The model under review builds one solid part; all positions refer to its coordinate system, in mm. A direction names the side the tool comes from. Give positions to 0.01 mm unless a question says otherwise; leave off trailing zeros. Order: outer loops, then holes, each group sorted by start corner. A loop starts at its lowest first (then second) coordinate and runs counter-clockwise, first axis right, second up. Notation, with made-up numbers: (58.5, 8) - (66.5, 8) arc R20 ccw to (66.5, 25) - close; hole circle Ø5 at (-19.5, -37). An arc over 180 degrees is marked (long way). Answer as CSV lines item,"result". Start each with the question number.
from build123d import *

# Parameters (mm, degrees)
SKIZZE1_W                       = 89
SKIZZE1_H                       = 71.5
LINEAR_AUSTRAGEN1_DEPTH         = 46
SKIZZE12_W                      = 89
SKIZZE12_H                      = 40.19389994
LINEAR_AUSTRAGEN2_DEPTH         = 45
LINEAR_AUSTRAGEN3_DEPTH         = 25
LINEAR_AUSTRAGEN9_DEPTH         = 1.5
SCHNITT_LINEAR_AUSTRAGEN1_DEPTH = 0.5
SKIZZE3_R                       = 1.5
SKIZZE3_R_2                     = 2.15
SKIZZE3_R_3                     = 3.2
LINEAR_AUSTRAGEN4_DEPTH         = 47
SKIZZE4_R                       = 4
SKIZZE4_R_2                     = 5.5
LINEAR_AUSTRAGEN5_DEPTH         = 6.5
SKIZZE13_R                      = 2.5
LINEAR_AUSTRAGEN8_DEPTH         = 8
SKIZZE10_R                      = 3.15
LINEAR_AUSTRAGEN6_DEPTH         = 28.3
SKIZZE11_R                      = 5.5
LINEAR_AUSTRAGEN7_DEPTH         = 23.3
LINEAR_AUSTRAGEN10_DEPTH        = 71.5


with BuildPart() as part:
    # Skizze1 → Linear austragen1 (new body)
    with BuildSketch(Plane.XY):
        with Locations((-3, 35.75)):
            Rectangle(SKIZZE1_W, SKIZZE1_H)
    extrude(amount=LINEAR_AUSTRAGEN1_DEPTH)

    # Skizze12 → Linear austragen2 (cut)
    with BuildSketch(Plane(origin=(0, 71.5, 0), x_dir=(1, 0, 0), z_dir=(0, 1, 0))):
        with Locations((-3, -32.09694997)):
            Rectangle(SKIZZE12_W, SKIZZE12_H)
    extrude(amount=-LINEAR_AUSTRAGEN2_DEPTH, mode=Mode.SUBTRACT)

    # Skizze2 → Linear austragen3 (cut)
    with BuildSketch(Plane.XZ.offset(-26.5)):
        with BuildLine():
            Line((-43.15, 46), (37.15, 46))
            Line((37.15, 46), (37.15, 44.3))
            ThreePointArc((37.15, 44.3), (36.388795325, 40.473165676), (34.221067812, 37.228932188))
            Line((34.221067812, 37.228932188), (28.221067812, 31.228932188))
            ThreePointArc((28.221067812, 31.228932188), (24.976834324, 29.061204675), (21.15, 28.3))
            Line((21.15, 28.3), (-27.15, 28.3))
            ThreePointArc((-27.15, 28.3), (-30.976834324, 29.061204675), (-34.221067812, 31.228932188))
            Line((-34.221067812, 31.228932188), (-40.221067812, 37.228932188))
            ThreePointArc((-40.221067812, 37.228932188), (-42.388795325, 40.473165676), (-43.15, 44.3))
            Line((-43.15, 44.3), (-43.15, 46))
        make_face()
    extrude(amount=LINEAR_AUSTRAGEN3_DEPTH, mode=Mode.SUBTRACT)

    # Skizze14 → Linear austragen9 (cut)
    with BuildSketch(Plane(origin=(0, 1.5, 0), x_dir=(-1, 0, 0), z_dir=(0, 1, 0))):
        with BuildLine():
            Line((13.462912018, 36.3), (33.15, 36.3))
            ThreePointArc((33.15, 36.3), (38.806854249, 38.643145751), (41.15, 44.3))
            Line((41.15, 44.3), (41.15, 46))
            Line((41.15, 46), (-35.15, 46))
            Line((-35.15, 46), (-35.15, 44.3))
            ThreePointArc((-35.15, 44.3), (-32.806854249, 38.643145751), (-27.15, 36.3))
            Line((-27.15, 36.3), (-13.462912018, 36.3))
            ThreePointArc((-13.462912018, 36.3), (0, 33.8), (13.462912018, 36.3))
        make_face()
    extrude(amount=-LINEAR_AUSTRAGEN9_DEPTH, mode=Mode.SUBTRACT)

    # Skizze16 → Schnitt-Linear austragen1 (cut)
    with BuildSketch(Plane(origin=(0, 1.5, 0), x_dir=(1, 0, 0), z_dir=(0, 1, 0))):
        with BuildLine():
            Line((21.15, -28.3), (-27.15, -28.3))
            ThreePointArc((-27.15, -28.3), (-30.976834324, -29.061204675), (-34.221067812, -31.228932188))
            Line((-34.221067812, -31.228932188), (-40.221067812, -37.228932188))
            ThreePointArc((-40.221067812, -37.228932188), (-41.635281374, -40.057359313), (-41.069595949, -43.16862915))
            ThreePointArc((-41.069595949, -43.16862915), (-38.391613931, -38.25636836), (-33.15, -36.3))
            Line((-33.15, -36.3), (-13.462912018, -36.3))
            ThreePointArc((-13.462912018, -36.3), (0, -33.8), (13.462912018, -36.3))
            Line((13.462912018, -36.3), (27.15, -36.3))
            ThreePointArc((27.15, -36.3), (32.391613931, -38.25636836), (35.069595949, -43.16862915))
            ThreePointArc((35.069595949, -43.16862915), (35.635281374, -40.057359313), (34.221067812, -37.228932188))
            Line((34.221067812, -37.228932188), (28.221067812, -31.228932188))
            ThreePointArc((28.221067812, -31.228932188), (24.976834324, -29.061204675), (21.15, -28.3))
        make_face()
    extrude(amount=-SCHNITT_LINEAR_AUSTRAGEN1_DEPTH, mode=Mode.SUBTRACT)

    # Skizze3 → Linear austragen4 (cut, through all)
    with BuildSketch(Plane(origin=(0, 0, 0), x_dir=(-1, 0, 0), z_dir=(0, 0, -1))):
        with Locations((15, 39)):
            Circle(SKIZZE3_R)
        with Locations((-15, 39)):
            Circle(SKIZZE3_R)
        with Locations((25, 64)):
            Circle(SKIZZE3_R_2)
        with Locations((-25, 64)):
            Circle(SKIZZE3_R_3)
    extrude(amount=-LINEAR_AUSTRAGEN4_DEPTH, mode=Mode.SUBTRACT)

    # Skizze4 → Linear austragen5 (cut)
    with BuildSketch(Plane(origin=(0, 0, 12), x_dir=(-1, 0, 0), z_dir=(0, 0, -1))):
        with Locations((25, 64)):
            Circle(SKIZZE4_R)
        with Locations((-25, 64)):
            Circle(SKIZZE4_R_2)
    extrude(amount=LINEAR_AUSTRAGEN5_DEPTH, mode=Mode.SUBTRACT)

    # Skizze13 → Linear austragen8 (cut)
    with BuildSketch(Plane.XY.offset(12)):
        with Locations((15, 39)):
            Circle(SKIZZE13_R)
        with Locations((-15, 39)):
            Circle(SKIZZE13_R)
    extrude(amount=-LINEAR_AUSTRAGEN8_DEPTH, mode=Mode.SUBTRACT)

    # Skizze10 → Linear austragen6 (cut)
    with BuildSketch(Plane(origin=(0, 0, 0), x_dir=(-1, 0, 0), z_dir=(0, 0, -1))):
        with Locations((0, 9.5)):
            Circle(SKIZZE10_R)
    extrude(amount=-LINEAR_AUSTRAGEN6_DEPTH, mode=Mode.SUBTRACT)

    # Skizze11 → Linear austragen7 (cut)
    with BuildSketch(Plane(origin=(0, 0, 0), x_dir=(-1, 0, 0), z_dir=(0, 0, -1))):
        with Locations((0, 9.5)):
            Circle(SKIZZE11_R)
    extrude(amount=-LINEAR_AUSTRAGEN7_DEPTH, mode=Mode.SUBTRACT)

    # Skizze15 → Linear austragen10 (cut)
    with BuildSketch(Plane.XZ):
        with BuildLine():
            Line((41.5, 44.3), (41.5, 0))
            Line((41.5, 0), (32.5, 0))
            Line((32.5, 0), (32.5, 24.737554159))
            ThreePointArc((32.5, 24.737554159), (33.41344561, 29.329755348), (36.014718626, 33.222835534))
            Line((36.014718626, 33.222835534), (37.545941546, 34.754058454))
            ThreePointArc((37.545941546, 34.754058454), (40.472373689, 39.133773663), (41.5, 44.3))
        make_face()
        with BuildLine():
            Line((-47.5, 44.3), (-47.5, 0))
            Line((-47.5, 0), (-40, 0))
            Line((-40, 0), (-40, 26.237554159))
            ThreePointArc((-40, 26.237554159), (-40.91344561, 30.829755348), (-43.514718626, 34.722835534))
            Line((-43.514718626, 34.722835534), (-43.545941546, 34.754058454))
            ThreePointArc((-43.545941546, 34.754058454), (-46.472373689, 39.133773663), (-47.5, 44.3))
        make_face()
    extrude(amount=-LINEAR_AUSTRAGEN10_DEPTH, mode=Mode.SUBTRACT)


solid = part.part
Item 1: Take a section at B-B on y = 64. Write out the cut boundary in (x, z).
Item 2: For line 1 along Y through (x, z) = (35, 35.5); line 2 along Y through (x, z) = (0, 25.8); line 3 along X through (y, z) = (52, 3.5), list the stretches that pass through material, from the lowest coordinate up.
Item 3: Mouldability with a two-part tool opening along X and no side actions: class faces 5 (the face through (-4, 71.5, 6)), 6 (the face through (-3, 14, 28.3)), 7 (the face through (33.4, 13.1, 29.3)) as released by +X, released by -X, zero draft, split by the parting line, or undercut.
Item 4: Machinability: for faces 1 (the face through (-42, 1.5, 44)), 2 (the face through (-40.9, 13.1, 30.8)), 3 (the face through (-4, 26.5, 21)), 4 (the face through (22.6, 61.6, 5.5)), which of the approach directions +Z, -Z, +X, -X, +Y, -Y give a long, thin tool a straight path to every point of the face, cutting with its end or side? Answer none if there is none.
Item 5: Take a section at A-A on x = -25. Write out the cut boundary in (y, z).
Item 6: Clearance check with flat-ended pins moving along their axes: pin 1 (3 mm diameter, centred on x = 35.5, z = 42, fed in from +Y); pin 2 (10 mm diameter, centred on y = 25.5, z = 33.5, fed in from +X); pin 3 (3.5 mm diameter, centred on x = -15, y = 39, fed in from +Z). State where each tip first meets the part, or that it passes through.
Item 7: Take a section at D-D on z = 7.5. Write out the cut boundary in (x, y), and give its area (3 significant figures).
Data:
1,outline,"(-40, 0) - (-27.15, 0) - (-27.15, 5.5) - (-29, 5.5) - (-29, 12) - (-40, 12) - close; (-22.85, 0) - (21.8, 0) - (21.8, 5.5) - (19.5, 5.5) - (19.5, 12) - (-21, 12) - (-21, 5.5) - (-22.85, 5.5) - close; (28.2, 0) - (32.5, 0) - (32.5, 12) - (30.5, 12) - (30.5, 5.5) - (28.2, 5.5) - close"
2,line 1,"y = 0 to 26.5"
2,line 2,"y = 0 to 6.35, 12.65 to 26.5"
2,line 3,"x = -40 to 32.5"
3,face 5,"zero draft"
3,face 6,"undercut"
3,face 7,"released by +X"
4,face 1,"+Z, +Y"
4,face 2,"-Z, -X, +Y, -Y"
4,face 3,"+Z, +X, -X, +Y"
4,face 4,"+Z"
5,outline,"(0, 0) - (61.85, 0) - (61.85, 5.5) - (60, 5.5) - (60, 12) - (26.5, 12) - (26.5, 28.3) - (1, 28.3) - (1, 36.3) - (0, 36.3) - close; (66.15, 0) - (71.5, 0) - (71.5, 12) - (68, 12) - (68, 5.5) - (66.15, 5.5) - close"
6,pin 1,"stops at y = 26.5"
6,pin 2,"stops at x = 40.19"
6,pin 3,"stops at z = 4"
7,outline,"(-40, 0) - (32.5, 0) - (32.5, 71.5) - (-40, 71.5) - close; hole circle Ø8 at (-25, 64); hole circle Ø5 at (-15, 39); hole circle Ø11 at (0, 9.5); hole circle Ø5 at (15, 39); hole circle Ø11 at (25, 64)"
7,area,"4,900 mm^2"
